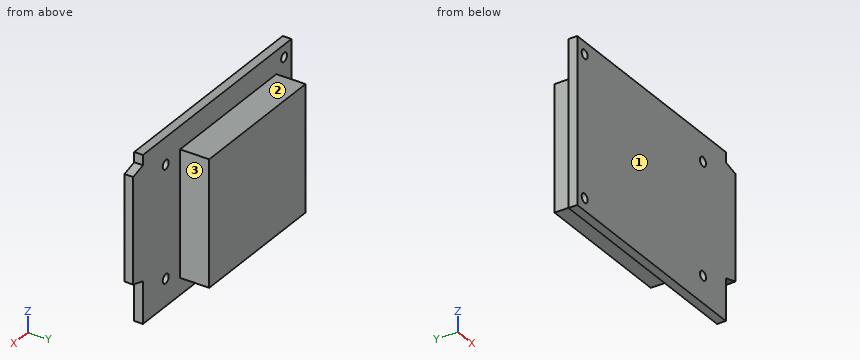
Autodesk Inventor part; units mm, degrees
ref_plane "YZ Plane" through (0, 0, 0) normal (1, 0, 0) x (0, 1, 0)
ref_plane "XZ Plane" through (0, 0, 0) normal (0, 1, 0) x (-1, 0, 0)
ref_plane "XY Plane" through (0, 0, 0) normal (0, 0, 1) x (1, 0, 0)
sketch "Sketch1" plane through (0, 0, 0) normal (0, 1, 0) x (-1, 0, 0)
  line L0 (0, 0) -> (-78.3209, 0)
  line L1 (-78.3209, 0) -> (-78.3209, -57.3913)
  line L2 (-78.3209, -57.3913) -> (0, -57.3913)
  line L3 (0, -57.3913) -> (0, 0)
  line L4 (-78.3209, -3.4798) -> (-78.3209, -42.8625)
  line L5 (-83.4511, -4.9086) -> (-83.4511, -41.4338)
  line L6 (-78.3209, -3.4798) -> (-83.4511, -4.9086)
  line L7 (-83.4511, -41.4338) -> (-78.3209, -42.8625)
  line L8 (-78.3209, -57.3913) -> (-78.3209, -42.8625)
  dimension "d0" = 78.3209
  dimension "d1" = 57.3913
  dimension "d2" = 39.3827
  dimension "d3" = 36.5252
  dimension "d4" = 14.5288
  dimension "d5" = 5.1303
extrude "Extrusion1" add sketch "Sketch1" along normal blind 3.048
sketch "Sketch2" plane through (0, 3.048, 0) normal (0, 1, 0) x (1, 0, 0)
  line L0 (78.3209, 57.3913) -> (0, 57.3913)
  line L1 (0, 57.3913) -> (2.3114, 57.3913)
  line L2 (2.3114, 57.3913) -> (2.3114, 54.6862)
  line L3 (2.3114, 54.6862) -> (0, 54.6862)
  line L4 (0, 54.6862) -> (0, 57.3913)
  line L5 (2.3114, 54.6862) -> (5.4864, 54.6862)
  line L6 (5.4864, 54.6862) -> (5.4864, 51.5874)
  line L7 (5.4864, 51.5874) -> (2.3114, 51.5874)
  line L8 (2.3114, 51.5874) -> (2.3114, 54.6862)
  circle A0 centre (3.8608, 53.1368) radius 1.5494
  line L9 (0, 57.3913) -> (0, 0)
  line L10 (0, 28.6957) -> (25.4, 28.6957)
  circle A1 centre (3.8608, 4.2545) radius 1.5494
  line L11 (0, 0) -> (78.3209, 0)
  line L12 (78.3209, 0) -> (67.8815, 0)
  line L13 (67.8815, 0) -> (67.8815, 57.3913)
  line L14 (67.8815, 57.3913) -> (78.3209, 57.3913)
  line L15 (78.3209, 57.3913) -> (78.3209, 0)
  line L16 (67.8815, 57.3913) -> (67.8815, 49.6443)
  line L17 (67.8815, 0) -> (67.8815, 7.747)
  line L18 (67.8815, 7.747) -> (64.7065, 7.747)
  line L19 (64.7065, 7.747) -> (64.7065, 10.922)
  line L20 (64.7065, 10.922) -> (67.8815, 10.922)
  line L21 (67.8815, 10.922) -> (67.8815, 7.747)
  line L22 (67.8815, 49.6443) -> (64.7065, 49.6443)
  line L23 (64.7065, 49.6443) -> (64.7065, 46.4693)
  line L24 (64.7065, 46.4693) -> (67.8815, 46.4693)
  line L25 (67.8815, 46.4693) -> (67.8815, 49.6443)
  circle A2 centre (66.294, 9.3345) radius 1.5875
  circle A3 centre (66.294, 48.0568) radius 1.5875
  dimension "d8" = 2.3114
  dimension "d9" = 2.7051
  dimension "d10" = 3.175
  dimension "d11" = 3.0988
  dimension "d12" = 10.4394
  dimension "d13" = 7.747
  dimension "d14" = 7.747
  dimension "d15" = 3.175
  dimension "d16" = 3.175
  dimension "d17" = 3.175
  dimension "d18" = 3.175
extrude "Extrusion2" cut sketch "Sketch2" against normal blind 3.048 contours A3 | A0 | A2 | A1
sketch "Sketch3" plane through (0, 3.048, 0) normal (0, 1, 0) x (1, 0, 0)
  line L0 (7.9375, 51.5874) -> (58.7375, 51.5874)
  line L1 (58.7375, 51.5874) -> (58.7375, 7.9375)
  line L2 (58.7375, 7.9375) -> (7.9375, 7.9375)
  line L3 (7.9375, 7.9375) -> (7.9375, 51.5874)
  point P0 (0, 0)
extrude "Extrusion3" add sketch "Sketch3" along normal blind 10.16
sketch "Sketch4" plane through (0, 0, 0) normal (0, -1, 0) x (1, 0, 0)
  line L0 (78.3209, -57.3913) -> (0, -57.3913)
  line L1 (0, 0) -> (78.3209, 0)
  line L2 (78.3209, 0) -> (78.3209, -57.3913)
  line L3 (78.3209, -57.3913) -> (0, -57.3913)
  line L4 (0, -57.3913) -> (0, 0)
  line L5 (0, 0) -> (78.3209, 0)
  line L6 (39.1604, 0) -> (39.1604, -57.3913)
  line L7 (78.3209, -28.6957) -> (0, -28.6957)
  line L8 (0, -57.3913) -> (0, 0)
sketch "Sketch5" plane through (0, 0, 0) normal (0, -1, 0) x (1, 0, 0)
  line L0 (39.1604, 0) -> (39.1604, -57.3913)
  line L1 (78.3209, -28.6957) -> (0, -28.6957)
  circle A0 centre (3.8608, -53.1368) radius 1.5494
  line L2 (39.1604, -28.6957) -> (3.8608, -28.6957)
  line L3 (3.8608, -28.6957) -> (3.8608, -53.1368)
  line L4 (3.8608, -53.1368) -> (39.1604, -53.1368)
  line L5 (39.1604, -53.1368) -> (39.1604, -28.6957)
  circle A1 centre (3.8608, -4.2545) radius 1.5494
  line L6 (39.1604, -28.6957) -> (3.8608, -28.6957)
  line L7 (3.8608, -28.6957) -> (3.8608, -4.2545)
  line L8 (3.8608, -4.2545) -> (39.1604, -4.2545)
  line L9 (39.1604, -4.2545) -> (39.1604, -28.6957)
  circle A2 centre (66.294, -9.3345) radius 1.5875
  line L10 (39.1604, -28.6957) -> (66.294, -28.6957)
  line L11 (66.294, -28.6957) -> (66.294, -9.3345)
  line L12 (66.294, -9.3345) -> (39.1604, -9.3345)
  line L13 (39.1604, -9.3345) -> (39.1604, -28.6957)
  circle A3 centre (66.294, -48.0568) radius 1.5875
  line L14 (39.1604, -28.6957) -> (66.294, -28.6957)
  line L15 (66.294, -28.6957) -> (66.294, -48.0568)
  line L16 (66.294, -48.0568) -> (39.1604, -48.0568)
  line L17 (39.1604, -48.0568) -> (39.1604, -28.6957)
  point P0 (0, 0)
  dimension "d23" = 24.4412
  dimension "d24" = 24.4412
  dimension "d25" = 35.2996
  dimension "d26" = 35.2996
  dimension "d27" = 27.1335
  dimension "d28" = 27.1335
  dimension "d29" = 19.3611
  dimension "d30" = 19.3611
properties part number "ProArduino"
Source: CAD feature listing. Evaluate the final solid. Frame: model axes, mm. Face numbers are marked on the shaded views. A direction names the side the tool comes from. Round coordinates to 2 decimals unless told otherwise and drop trailing zeros. Loops run counter-clockwise (first coordinate to the right, second up) from the corner with the lowest first, then second, coordinate; pieces in that order, holes last. Notation, with made-up numbers: (-40, 63) - (-6, 63) arc R37 cw to (-6, 99) - close; hole circle Ø11 at (-34.5, 0). An arc over 180 degrees is marked (long way). Write item = value, one per line. Start each with the question number.
Item 1: Section query C-C on y = 1.75. Output: boundary loops of the cut face in (x, z) (1 decimal).
Item 2: Section query D-D on x = 72. Output: boundary loops of the cut face in (y, z), plus the area to 3 significant figures.
Item 3: First-contact query: pin 1 Ø6 at (x, y) = (24, 11) entering from -Z; pin 2 Ø2 at (y, z) = (5, -33) entering from +X; pin 3 Ø3.5 at (y, z) = (1.5, -52.5) entering from +X; pin 4 Ø6 at (x, z) = (18, -35) entering from -Y. Flat tips, straight axial feed; report the tip coordinate or a pass-through.
Item 4: Material intervals for line 1 (X direction, y = 2, z = -54); line 2 (X direction, y = 9.5, z = -37); line 3 (Y direction, x = 60.5, z = -21.5), sorted ascending.
Item 5: Section query A-A on z = -23.5. Output: boundary loops of the cut face in (x, y), plus the area to 3 significant figures.
Item 6: Reachability of the marked faces 1, 2 and 3 from +Z, -Z, +X, -X, +Y, -Y: full face, straight path, thin tool, end or side. Return the list, or none.
Item 7: Section query B-B on x = 48. Output: boundary loops of the cut face in (y, z).
Results list:
q1.outline = (0, -57.4) - (78.3, -57.4) - (78.3, -42.9) - (83.5, -41.4) - (83.5, -4.9) - (78.3, -3.5) - (78.3, 0) - (0, 0) - close; hole circle Ø3.1 at (3.9, -53.1); hole circle Ø3.1 at (3.9, -4.3); hole circle Ø3.2 at (66.3, -48.1); hole circle Ø3.2 at (66.3, -9.3)
q2.outline = (0, -57.39) - (3.05, -57.39) - (3.05, 0) - (0, 0) - close
q2.area = 175 mm²
q3.pin_1 = -51.59
q3.pin_2 = 58.74
q3.pin_3 = 78.32
q3.pin_4 = 0
q4.line_1 = 0 to 2.57, 5.15 to 78.32
q4.line_2 = 7.94 to 58.74
q4.line_3 = 0 to 3.05
q5.outline = (0, 0) - (83.45, 0) - (83.45, 3.05) - (58.74, 3.05) - (58.74, 13.21) - (7.94, 13.21) - (7.94, 3.05) - (0, 3.05) - close
q5.area = 770 mm²
q6.face_1 = +Z, -Z, +X, -X, -Y
q6.face_2 = +Z, +X, -X, +Y
q6.face_3 = +Z, -Z, +X, +Y
q7.outline = (0, -57.39) - (3.05, -57.39) - (3.05, -51.59) - (13.21, -51.59) - (13.21, -7.94) - (3.05, -7.94) - (3.05, 0) - (0, 0) - close
